```python
from build123d import *

# Parameters (mm, degrees)
F0_W       = 875
F0_H       = 303
F1_DEPTH   = 22
F2_SIZE2   = 8.007335
F2_SIZE    = 21.99999
F2_2_SIZE2 = 8.007335
F2_2_SIZE  = 21.99999
F3_W       = 25
F3_H       = 16
F4_DEPTH   = 200


# Not quite as in the source:
# - a fillet or chamfer is up to 0.001 mm smaller than in the source, because OpenCascade refuses the exact size


with BuildPart() as f1:
    # F0 (on Front) → F1 (new body)
    with BuildSketch(Plane.XZ):
        Rectangle(F0_W, F0_H)
    extrude(amount=F1_DEPTH)

    # F2 (size 22 and 8.0073451539 in the source; OpenCascade refuses exactly that, so slightly less here)
    f2_edges = [f1.edges().sort_by_distance(p)[0] for p in [
        (0, -22, -151.5),
    ]]
    f2_side = f1.faces().sort_by_distance((0, -11, -151.5))[0]
    chamfer(f2_edges, length=F2_SIZE, length2=F2_SIZE2, reference=f2_side)

    # F2#2 (size 22 and 8.0073451539 in the source; OpenCascade refuses exactly that, so slightly less here)
    f2_2_edges = [f1.edges().sort_by_distance(p)[0] for p in [
        (0, 0, 151.5),
    ]]
    f2_2_side = f1.faces().sort_by_distance((0, -11, 151.5))[0]
    chamfer(f2_2_edges, length=F2_2_SIZE, length2=F2_2_SIZE2, reference=f2_2_side)

    # F3 (on Top) → F4 (cut, symmetric)
    with BuildSketch(Plane.XY):
        with Locations((425, -8)):
            Rectangle(F3_W, F3_H)
        with Locations((-425, -8)):
            Rectangle(F3_W, F3_H)
    extrude(amount=F4_DEPTH, both=True, mode=Mode.SUBTRACT)


solid = f1.part
```
Model file for the job. Use its own axes, mm. A direction names the side the tool comes from. Round coordinates to 2 decimals unless told otherwise and drop trailing zeros. Order: outer loops, then holes, each group sorted by start corner. A loop starts at its lowest first (then second) coordinate and runs counter-clockwise, first axis right, second up. Notation, with made-up numbers: M 2.25,26.25 L 12.25,26.25 A12 ccw 12.25,30.25 Z; hole C 89,73.25 d2. An arc over 180 degrees is marked long. Use CSV: the item, a comma, the result in double quotes.
Item 1: Saw through at A-A (z = 122.5). List the corners of the cut face in (x, y).
Worked answers:
outline,"M -437.5,-22 L 437.5,-22 L 437.5,-16 L 412.5,-16 L 412.5,0 L -412.5,0 L -412.5,-16 L -437.5,-16 Z"
Item 2: Pin check, flat tips, straight feed: pin 1 (1 mm diameter, centred on x = 110.5, y = -11, fed in from +Z); pin 2 (7.5 mm diameter, centred on x = -430, z = -40, fed in from +Y); pin 3 (8 mm diameter, centred on y = -5.5, z = 4, fed in from -X). Stop position of each tip, or through.
Worked answers:
pin 1,"z = 147.68"
pin 2,"y = -16"
pin 3,"x = -412.5"
Item 3: Which spindle directions (+Z, -Z, +X, -X, +Y, -Y) get a long thin tool onto all of the face, cutting with end or side? Do faces 1 (the face through (-425, -16, 4)), 2 (the face through (-6, 0, -2)), 3 (the face through (425, -16, 0)). Say none if no direction does.
Worked answers:
face 1,"+Z, -Z, -X, +Y"
face 2,"+Z, -Z, +X, -X, +Y"
face 3,"+Z, -Z, +X, +Y"
Item 4: Saw through at C-C (y = -11.25). List the corners of the cut face in (x, z).
Worked answers:
outline,"M -412.5,-147.41 L 412.5,-147.41 L 412.5,147.59 L -412.5,147.59 Z"
Item 5: Probe probe 1 along X at (y, z) = (-1.75, -2); probe 2 along Z at (x, y) = (321, -10.25); probe 3 along Z at (x, y) = (-3.5, -8.75). List the from-to ranges inside material, lowest first.
Worked answers:
probe 1,"-412.5 to 412.5"
probe 2,"-147.77 to 147.22"
probe 3,"-148.32 to 146.68"
